```python
from build123d import *

# Parameters (mm, degrees)
SKETCH_1_R      = 0.5
EXTRUDE_1_DEPTH = 150
FILLET_1_R      = 0.3


with BuildPart() as part:
    # 草图1 → 凸台-拉伸1 (new body)
    with BuildSketch(Plane.XY):
        with BuildLine():
            Line((18, 1), (0, 1))
            ThreePointArc((0, 1), (-1, 0), (0, -1))
            Line((0, -1), (18, -1))
            Line((18, -1), (18, 1))
        make_face()
        Circle(SKETCH_1_R, mode=Mode.SUBTRACT)
    extrude(amount=EXTRUDE_1_DEPTH)

    # 圆角1
    fillet_1_edges = [part.edges().sort_by_distance(p)[0] for p in [
        (18, 1, 75),
        (18, -1, 75),
    ]]
    fillet(fillet_1_edges, radius=FILLET_1_R)


solid = part.part
```
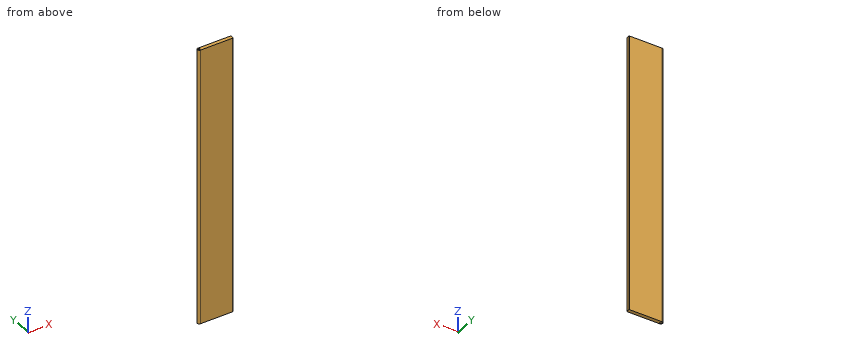
The listing builds one solid part. Answer for the finished solid, in the listing's coordinates (mm). Round coordinates to 2 decimals unless told otherwise and drop trailing zeros. Order: outer loops, then holes, each group sorted by start corner. A loop starts at its lowest first (then second) coordinate and runs counter-clockwise, first axis right, second up. Notation, with made-up numbers: (50.5, -9.75) - (93.5, -9.75) arc R19 ccw to (93.5, 11.25) - close; hole circle Ø3 at (56.25, 50.5). An arc over 180 degrees is marked (long way). Put each result on its own line as item: value. Start each with the question number.
(1) Straight lines are drawn through the part: probe 1 along Y at (x, z) = (0, 58.5); probe 2 along X at (y, z) = (-0.15, 98.5); probe 3 along X at (y, z) = (-0.4, 123.5). For each, find the intervals that lie inside material, in ascending order. Write a range as from..to.
(2) Find section B-B (z = 91). Give the vertices of the cut face in (x, y).
(3) Find section A-A (y = 0). Give the vertices of the cut face in (x, z), plus the area to 3 significant figures.
Reply:
1. probe 1: -1..-0.5, 0.5..1
1. probe 2: -0.99..-0.48, 0.48..18
1. probe 3: -0.92..-0.3, 0.3..18
2. outline: (0, -1) - (17.7, -1) arc R0.3 ccw to (18, -0.7) - (18, 0.7) arc R0.3 ccw to (17.7, 1) - (0, 1) arc R1 ccw to start; hole circle Ø1 at (0, 0)
3. outline: (-1, 0) - (-0.5, 0) - (-0.5, 150) - (-1, 150) - close; (0.5, 0) - (18, 0) - (18, 150) - (0.5, 150) - close
3. area: 2,700 mm^2
